```python
from build123d import *

# Parameters (mm, degrees)
SKETCH1_R           = 51.838
SKETCH1_R_2         = 50.822
BOSS_EXTRUDE1_DEPTH = 54
CUT_EXTRUDE1_DEPTH  = 53
CUT_EXTRUDE2_START  = -1
SKETCH3_R           = 51.838
SKETCH3_R_2         = 50.822
CUT_EXTRUDE2_DEPTH  = 1


with BuildPart() as part:
    # Sketch1 → Boss-Extrude1 (new body)
    with BuildSketch(Plane(origin=(0, 0, 0), x_dir=(1, 0, 0), z_dir=(0, 1, 0))):
        with Locations(Location((-43.858802719, -17.175645915, 0), (0, 0, 270))):
            Circle(SKETCH1_R)
        with Locations(Location((-43.858802719, -17.175645915, 0), (0, 0, 270))):
            Circle(SKETCH1_R_2, mode=Mode.SUBTRACT)
    extrude(amount=BOSS_EXTRUDE1_DEPTH)

    # Sketch2 → Cut-Extrude1 (cut)
    with BuildSketch(Plane.XY):
        with BuildLine():
            Line((-56.540802719, 20.5), (-56.540802719, -11.133422885))
            Line((-56.540802719, -11.133422885), (-31.176802719, -11.133422885))
            Line((-31.176802719, -11.133422885), (-31.176802719, 20.5))
            ThreePointArc((-31.176802719, 20.5), (-43.858802719, 33.182), (-56.540802719, 20.5))
        make_face()
    extrude(amount=-CUT_EXTRUDE1_DEPTH, mode=Mode.SUBTRACT)

    # Sketch3 → Cut-Extrude2 (cut)
    with BuildSketch(Plane(origin=(0, 54, 0), x_dir=(1, 0, 0), z_dir=(0, 1, 0)).offset(CUT_EXTRUDE2_START)):
        with Locations(Location((-43.858802719, -17.175645915, 0), (0, 0, 75.839039259))):
            Circle(SKETCH3_R)
        with Locations(Location((-43.858802719, -17.175645915, 0), (0, 0, 75.54984846))):
            Circle(SKETCH3_R_2, mode=Mode.SUBTRACT)
    extrude(amount=CUT_EXTRUDE2_DEPTH, mode=Mode.SUBTRACT)


solid = part.part
```
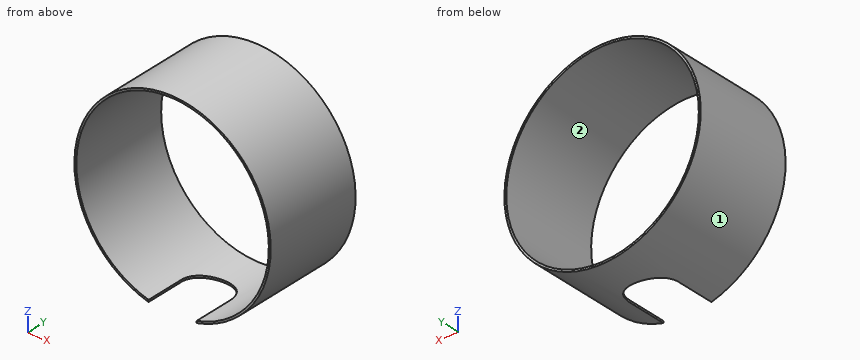
Here's how the part is built. I have some questions about the finished solid (model axes, mm). Face numbers are marked on the shaded views. Round coordinates to 2 decimals unless told otherwise and drop trailing zeros. Write each loop counter-clockwise with the first axis right and the second up, starting at its lowest first coordinate (ties: lowest second). Pieces come first, ordered by that corner, then holes.
Q1. If we section it at B-B on z = 38.5: Write out the boundary of the cut face in (x, y), plus the area to 3 significant figures.
Q2. If we mould it in two halves opening along Z, with no side actions, what happens to the marked faces 1 and 2? For each: +Z half, -Z half, draft (parallel to the pull), parting line (faces both ways), or undercut.
Q3. If we section it at C-C on y = 38.5: Write out the boundary of the cut face in (x, z).
Q4. If we section it at D-D on y = 25: Write out the boundary of the cut face in (x, z).
Q5. Please list where these lines run through material, in increasing order: probe 1 along X at (y, z) = (18.5, 17.5); probe 2 along X at (y, z) = (21, -17); probe 3 along Z at (x, y) = (-43, 49).
Q6. If we section it at A-A on x = -88: Write out the boundary of the cut face in (y, z), plus the area to 3 significant figures.
Q7. Will these pins go through, and if not, where does the flat tip stop? P1, Ø8, axis at x = -12.5, y = 7.5, coming from the -Z side; P2, Ø6, axis at x = -55, y = 44.5, coming from the -Z side; P3, Ø3, axis at y = 17.5, z = -12.5, coming from the -X side.
Answer below:
1. outline: (-91.11, 0) - (-89.99, 0) - (-89.99, 53) - (-91.11, 53) - close; (2.27, 0) - (3.39, 0) - (3.39, 53) - (2.27, 53) - close
1. area: 118 mm2
2. face 1: parting line
2. face 2: undercut
3. outline: circle Ø103.68 at (-43.86, 17.18); hole circle Ø101.64 at (-43.86, 17.18)
4. outline: (-55.72, -33.29) - (-55.72, -32.24) arc R50.82 cw (long way) to (-32, -32.24) - (-32, -33.29) arc R51.84 ccw (long way) to start
5. probe 1: x = -95.7 to -94.68, 6.96 to 7.98
5. probe 2: x = -82.84 to -81.47, -6.24 to -4.88
5. probe 3: z = -34.66 to -33.64, 67.99 to 69.01
6. outline: (0, -10) - (53, -10) - (53, -8.01) - (0, -8.01) - close; (0, 42.36) - (53, 42.36) - (53, 44.36) - (0, 44.36) - close
6. area: 211 mm2
7. P1: stops at z = -26.85
7. P2: stops at z = -34.02
7. P3: stops at x = -87.37
